Geometry check sheet. Reference: drawing and pictorial views, mm from the part's lowest x, y, z. A direction names the side the tool comes from. Round coordinates to 2 decimals unless told otherwise and drop trailing zeros. Order: outer loops, then holes, each group sorted by start corner. A loop starts at its lowest first (then second) coordinate and runs counter-clockwise, first axis right, second up.
(1) Tool access check on the marked faces 4, 5 and 6. Record the directions out of +Z, -Z, +X, -X, +Y, -Y that give a thin tool (end or side, any length) a straight path to the whole face; none if there is none.
(2) Sectioned sample at D-D, the plane y = 36. Enter the section's corners in (x, z), and give its area (3 significant figures).
(3) Mould release check, pull along X, two halves, no side actions. Record for the marked faces 1, 2 and 3: released by +X, released by -X, zero draft, split by the parting line, or undercut.
(4) Sectioned sample at A-A, the plane y = 51. Enter the section's corners in (x, z), and give its area (3 significant figures).
(5) Depth check by flat-ended pin: pin 1 (3 mm diameter, centred on x = 10, y = 51, fed in from +Z); pin 2 (3 mm diameter, centred on x = 11, z = 9, fed in from -Y); pin 3 (10 mm diameter, centred on x = 7, y = 36.5, fed in from +Z); pin 4 (12 mm diameter, centred on x = 16, z = 26, fed in from +Y). Enter the tip coordinate at first touch or a pass-through.
(6) Sectioned sample at B-B, the plane x = 10. Enter the section's corners in (y, z), and give its area (3 significant figures).
(7) Thickness scan on probe 1 along Y at (x, z) = (10, 2.6); probe 2 along Y at (x, z) = (10, 28); probe 3 along Y at (x, z) = (14.75, 23.5). Record the ranges inside material, lowest first.
(8) Sectioned sample at C-C, the plane x = 16.75. Enter the section's corners in (y, z), and give its area (3 significant figures).
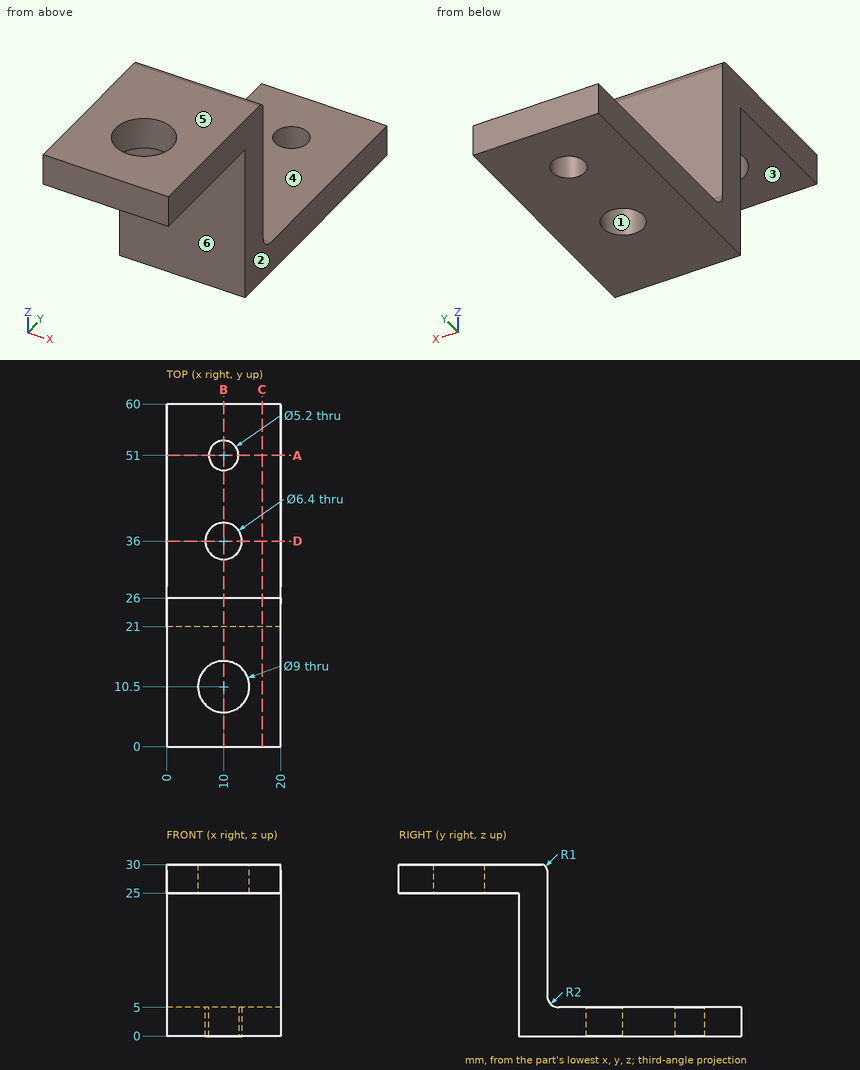
Derived:
1. face 4: +Z, +X, -X, +Y
1. face 5: +Z, +X, -X, +Y, -Y
1. face 6: -Z, +X, -X, -Y
2. outline: (0, 0) - (6.8, 0) - (6.8, 5) - (0, 5) - close; (13.2, 0) - (20, 0) - (20, 5) - (13.2, 5) - close
2. area: 68.0 mm2
3. face 1: undercut
3. face 2: released by +X
3. face 3: zero draft
4. outline: (0, 0) - (7.4, 0) - (7.4, 5) - (0, 5) - close; (12.6, 0) - (20, 0) - (20, 5) - (12.6, 5) - close
4. area: 74.0 mm2
5. pin 1: passes through
5. pin 2: stops at y = 21
5. pin 3: stops at z = 5
5. pin 4: stops at y = 26
6. outline: (0, 25) - (6, 25) - (6, 30) - (0, 30) - close; (15, 25) - (21, 25) - (21, 0) - (32.8, 0) - (32.8, 5) - (28, 5) arc R2 cw to (26, 7) - (26, 29) arc R1 ccw to (25, 30) - (15, 30) - close; (39.2, 0) - (48.4, 0) - (48.4, 5) - (39.2, 5) - close; (53.6, 0) - (60, 0) - (60, 5) - (53.6, 5) - close
6. area: 323 mm2
7. probe 1: y = 21 to 32.8, 39.2 to 48.4, 53.6 to 60
7. probe 2: y = 0 to 6, 15 to 26
7. probe 3: y = 21 to 26
8. outline: (0, 25) - (21, 25) - (21, 0) - (60, 0) - (60, 5) - (28, 5) arc R2 cw to (26, 7) - (26, 29) arc R1 ccw to (25, 30) - (0, 30) - close
8. area: 426 mm2
